Read the model definition and answer for the solid it produces. Units are mm, in the model's axes. Round coordinates to 2 decimals unless told otherwise and drop trailing zeros. Order: outer loops, then holes, each group sorted by start corner. A loop starts at its lowest first (then second) coordinate and runs counter-clockwise, first axis right, second up. Notation, with made-up numbers: (64, 17.5) -> (89, 17.5) arc R16 cw to (89, 44.5) -> close; hole circle Ø8 at (59, -28). An arc over 180 degrees is marked (long way). Answer as a JSON object with one key per item and string values. Group by question number.
Item 1: Section B-B, the plane y = 0 is taken. Write down the section's boundary in (x, z).
Item 2: Consider probe 1 along Y at (x, z) = (-17.5, 37.5); probe 2 along Y at (x, z) = (29, -26.5); probe 3 along Z at (x, y) = (-3, 40.5). Determine where each line is inside the solid, lowest interval first. Write a range as from..to.
Item 3: Given P1, Ø1, axis at y = 11.5, z = 15, coming from the +X side; P2, Ø5, axis at x = -24.5, y = 3, coming from the +Z side; P3, Ø3, axis at x = -31.242, y = 0, coming from the -Z side, each flat-ended and moving along its own axis, determine where each tip first touches the part or whether it passes through.
Item 4: Section D-D, the plane z = -24.5 is taken. Write down the section's boundary in (x, y), plus the area to 3 significant figures.
Item 5: Section C-C, the plane z = 0 is taken. Write down the section's boundary in (x, y), plus the area to 3 significant figures.
Item 6: Section A-A, the plane x = 0 is taken. Write down the section's boundary in (y, z).
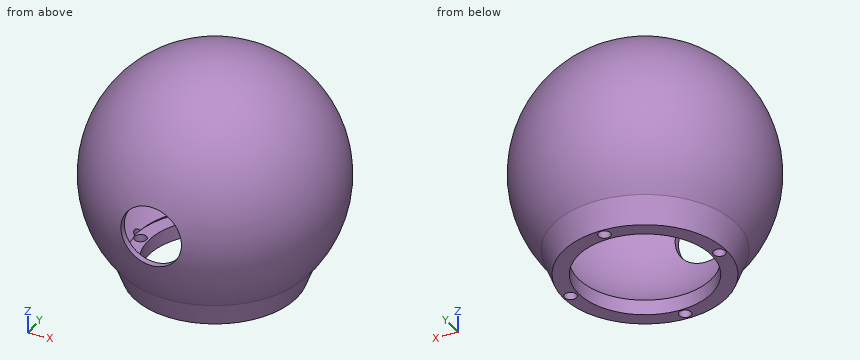
from build123d import *

# Parameters (mm, degrees)
F0_W     = 6.35
F0_H     = 6.35
F2_D     = 25.4
F2_DEPTH = 50.801
F4_D     = 5.08
F4_DEPTH = 43.832140591
F6_D     = 5.08
F6_DEPTH = 43.832140591
F7_D     = 5.08
F7_DEPTH = 43.832140591


with BuildPart() as f1:
    # F0 (on Front) → F1 (revolve)
    with BuildSketch(Plane.XZ):
        with BuildLine():
            ThreePointArc((38.401894824, -33.2555931225), (46.2061907682, 21.1099013425), (0, 50.8))
            Line((0, 50.8), (0, 48.26))
            ThreePointArc((0, 48.26), (44.9856946855, 17.4732616779), (32.5755, -35.6070835614))
            Line((32.5755, -35.6070835614), (34.29, -37.481140591))
            ThreePointArc((34.29, -37.481140591), (36.407302923, -35.4280721162), (38.401894824, -33.2555931225))
        make_face()
        with Locations((31.115, -40.656140591)):
            Rectangle(F0_W, F0_H)
        with BuildLine():
            Line((34.29, -43.831140591), (38.401894824, -33.2555931225))
            ThreePointArc((38.401894824, -33.2555931225), (36.407302923, -35.4280721162), (34.29, -37.481140591))
            Line((34.29, -37.481140591), (34.29, -43.831140591))
        make_face()
    revolve(axis=Axis((0, 0, 49.53), (0, 0, 1)))

    # F2 (through all, one way)
    with BuildSketch(Plane(origin=(0, 0, 0), x_dir=(1, 0, 0), z_dir=(0, 1, 0))):
        with Locations((0, 0)):
            Circle(F2_D / 2)
    extrude(amount=-F2_DEPTH, mode=Mode.SUBTRACT)

    # F4 (through all, one way)
    with BuildSketch(Plane.XY):
        with Locations((-31.242, 0)):
            Circle(F4_D / 2)
    extrude(amount=-F4_DEPTH, mode=Mode.SUBTRACT)

    # F6 (through all, one way)
    with BuildSketch(Plane.XY):
        with Locations((0, -30.988)):
            Circle(F6_D / 2)
    extrude(amount=-F6_DEPTH, mode=Mode.SUBTRACT)

    # F7 (through all, one way)
    with BuildSketch(Plane.XY):
        with Locations((0, 31.242), (31.242, 0)):
            Circle(F7_D / 2)
    extrude(amount=-F7_DEPTH, mode=Mode.SUBTRACT)


solid = f1.part
Values found:
{
 "1": {"outline": "(-38.4, -33.26) -> (-34.29, -43.83) -> (-33.78, -43.83) -> (-33.78, -37.48) -> (-34.29, -37.48) -> (-33.78, -36.93) -> (-33.78, -34.46) arc R48.26 cw (long way) to (33.78, -34.46) -> (33.78, -36.93) -> (34.29, -37.48) -> (33.78, -37.48) -> (33.78, -43.83) -> (34.29, -43.83) -> (38.4, -33.26) arc R50.8 ccw (long way) to start; (-28.7, -43.83) -> (-27.94, -43.83) -> (-27.94, -37.48) -> (-28.7, -37.48) -> close; (27.94, -43.83) -> (28.7, -43.83) -> (28.7, -37.48) -> (27.94, -37.48) -> close"},
 "2": {"probe 1": "-29.46..-24.83, 24.83..29.46", "probe 2": "-32.21..-28.03, 28.03..32.21", "probe 3": "-30.52..-26.07, 26.07..30.52"},
 "3": {"P1": "x = 47.35", "P2": "z = 45.7", "P3": "z = 35.45"},
 "4": {"outline": "circle Ø89 at (0, 0); hole circle Ø83.16 at (0, 0)", "area": "790 mm2"},
 "5": {"outline": "(-12.7, -49.19) -> (-12.7, -46.56) arc R48.26 cw (long way) to (12.7, -46.56) -> (12.7, -49.19) arc R50.8 ccw (long way) to start", "area": "725 mm2"},
 "6": {"outline": "(-49.19, -12.7) arc R50.8 ccw to (-38.4, -33.26) -> (-34.29, -43.83) -> (-33.53, -43.83) -> (-33.53, -37.48) -> (-34.29, -37.48) -> (-33.53, -36.65) -> (-33.53, -34.71) arc R48.26 cw to (-46.56, -12.7) -> close; (-49.19, 12.7) -> (-46.56, 12.7) arc R48.26 cw (long way) to (33.78, -34.46) -> (33.78, -36.93) -> (34.29, -37.48) -> (33.78, -37.48) -> (33.78, -43.83) -> (34.29, -43.83) -> (38.4, -33.26) arc R50.8 ccw (long way) to start; (-28.45, -43.83) -> (-27.94, -43.83) -> (-27.94, -37.48) -> (-28.45, -37.48) -> close; (27.94, -43.83) -> (28.7, -43.83) -> (28.7, -37.48) -> (27.94, -37.48) -> close"}
}
